Part model, mm, in its own coordinate system. A direction names the side the tool comes from. Round coordinates to 2 decimals unless told otherwise and drop trailing zeros. Order: outer loops, then holes, each group sorted by start corner. A loop starts at its lowest first (then second) coordinate and runs counter-clockwise, first axis right, second up. Notation, with made-up numbers: (88.5, -8.5) -> (136.5, -8.5) arc R14 cw to (136.5, 10.5) -> close; hole circle Ø10 at (-7, 51.5). An arc over 180 degrees is marked (long way). Use CSV: the item, a comma, the result in double quotes.
```python
from build123d import *

# Parameters (mm, degrees)
F0_W     = 38.1
F0_H     = 38.1
F1_DEPTH = 0.79375
F2_W     = 38.1
F2_H     = 38.1
F2_W_2   = 34.925
F2_H_2   = 34.925
F3_DEPTH = 6.35
F4_W     = 14.224
F4_H     = 1.898194
F4_W_2   = 2.502164
F4_H_2   = 2.067971
F4_W_3   = 5.951583
F4_H_3   = 0.006806
F4_W_4   = 18.415
F4_H_4   = 2.333408
F5_DEPTH = 4.445


with BuildPart() as f1:
    # F0 (on Top) → F1 (new body)
    with BuildSketch(Plane.XY):
        with Locations((-5.390748, 5.977843)):
            Rectangle(F0_W, F0_H)
    extrude(amount=F1_DEPTH)

    # F2 (on face) → F3 (join)
    with BuildSketch(Plane.XY.offset(0.79375)):
        with Locations((-5.390748, 5.977843)):
            Rectangle(F2_W, F2_H)
        with Locations((-5.390748, 5.977843)):
            Rectangle(F2_W_2, F2_H_2, mode=Mode.SUBTRACT)
    extrude(amount=F3_DEPTH)

    # F4 (on face) → F5 (join)
    with BuildSketch(Plane.XY.offset(0.79375)):
        Polygon((-17.773248, -11.484657), (-16.99117, -11.484657), (-16.503248, -11.484657), (-16.503248, 9.445464), (-17.773248, 9.445464), align=None)
        Polygon((-16.503248, 18.360343), (-16.99117, 18.360343), (-17.773248, 18.360343), (-17.773248, 17.845441), (-16.503248, 17.845441), align=None)
        Polygon((-16.503248, 17.845441), (-17.773248, 17.845441), (-17.773248, 16.637499), (-17.773248, 14.525464), (-16.503248, 14.525464), align=None)
        with Locations((-4.311248, 17.411246)):
            Rectangle(F4_W, F4_H)
        Polygon((6.991752, 18.360343), (2.800752, 18.360343), (2.800752, 16.462149), (2.800752, 11.375343), (6.991752, 11.375343), (6.991752, 14.394178), (6.991752, 16.462149), align=None)
        Polygon((6.991752, 11.375343), (2.800752, 11.375343), (-2.279248, 11.375343), (-8.230831, 11.375343), (-11.423248, 11.375343), (-11.423248, 6.295343), (6.991752, 6.295343), align=None)
        with Locations((8.242834, 15.428164)):
            Rectangle(F4_W_2, F4_H_2)
        with Locations((-5.25504, 11.378746)):
            Rectangle(F4_W_3, F4_H_3)
        Polygon((12.071752, 6.295343), (6.991752, 6.295343), (6.991752, 3.961935), (-11.423248, 3.961935), (-11.423248, -6.404657), (12.071752, -6.404657), align=None)
        with Locations((-2.215748, 5.128639)):
            Rectangle(F4_W_4, F4_H_4)
    extrude(amount=F5_DEPTH)


solid = f1.part
```
(1) Cut at B-B, the plane z = 6.5. Give the cut face in (x, y), then the cut area to 3 significant figures.
Reply:
outline,"(-24.44, -13.07) -> (13.66, -13.07) -> (13.66, 25.03) -> (-24.44, 25.03) -> close; hole (-22.85, -11.48) -> (12.07, -11.48) -> (12.07, 23.44) -> (-22.85, 23.44) -> close"
area,"232 mm2"
(2) Pull direction X, two halves, no side cores. Call faces 3 (the face through (-4, 16.462, 3)), 4 (the face through (-6, 6, 0)), 5 (the face through (0, -6.405, 3)): released by +X, released by -X, zero draft, split by the parting line, or undercut.
Reply:
face 3,"undercut"
face 4,"zero draft"
face 5,"undercut"
(3) Probe probe 1 along Y at (x, z) = (9, 2.75); probe 2 along X at (y, z) = (13, 1.5); probe 3 along Y at (x, z) = (3.5, 2.5). List the from-to ranges inside material, lowest first. Write a range as [from, to].
Reply:
probe 1,"[-13.07, -11.48], [-6.4, 6.3], [14.39, 16.46], [23.44, 25.03]"
probe 2,"[-24.44, -22.85], [2.8, 6.99], [12.07, 13.66]"
probe 3,"[-13.07, -11.48], [-6.4, 18.36], [23.44, 25.03]"
(4) Cut at D-D, the plane x = -3.5. Give the cut face in (y, z), then the cut area to 3 significant figures.
Reply:
outline,"(-13.07, 0) -> (25.03, 0) -> (25.03, 7.14) -> (23.44, 7.14) -> (23.44, 0.79) -> (18.36, 0.79) -> (18.36, 5.24) -> (16.46, 5.24) -> (16.46, 0.79) -> (11.38, 0.79) -> (11.38, 5.24) -> (-6.4, 5.24) -> (-6.4, 0.79) -> (-11.48, 0.79) -> (-11.48, 7.14) -> (-13.07, 7.14) -> close"
area,"138 mm2"
(5) Cut at A-A, the plane z = 4.25. State how many separate pieces and enclosed holes the cut face has, then the cut area to 3 significant figures.
Reply:
separate pieces,"2"
enclosed holes,"1"
area,"717 mm2"
(6) Drop flat-ended pins along their axis: P1, Ø6, axis at x = -18, y = 16.5, coming from the -Z side; P2, Ø1.4, axis at x = -17, y = 17, coming from the +Z side. Give the stop position or say it passes through.
Reply:
P1,"z = 0"
P2,"z = 5.24"
(7) Cut at C-C, the plane y = -8. Give the cut face in (x, z), then the cut area to 3 significant figures.
Reply:
outline,"(-24.44, 0) -> (13.66, 0) -> (13.66, 7.14) -> (12.07, 7.14) -> (12.07, 0.79) -> (-16.5, 0.79) -> (-16.5, 5.24) -> (-17.77, 5.24) -> (-17.77, 0.79) -> (-22.85, 0.79) -> (-22.85, 7.14) -> (-24.44, 7.14) -> close"
area,"56.0 mm2"
(8) Which spindle directions (+Z, -Z, +X, -X, +Y, -Y) get a long thin tool onto all of the face, cutting with end or side? Do faces 1 (the face through (2.801, 14, 3)), 2 (the face through (-6, -13.072, 4)). Say none if no direction does.
Reply:
face 1,"+Z"
face 2,"+Z, -Z, +X, -X, -Y"
